```python
from build123d import *

# Parameters (mm, degrees)
ESQUISSE1_W                = 250
ESQUISSE1_H                = 50
BOSS_EXTRU_1_DEPTH         = 3.175
ESQUISSE2_W                = 10
ESQUISSE2_H                = 3.175
BOSS_EXTRU_2_DEPTH         = 3.175
R_P_TITION_LIN_AIRE1_COUNT = 13
R_P_TITION_LIN_AIRE1_PITCH = 20
ESQUISSE4_W                = 40
ESQUISSE4_H                = 23
ESQUISSE4_W_2              = 20
ESQUISSE4_H_2              = 3.175
ENL_V_MAT_EXTRU_1_DEPTH    = 3.175
ESQUISSE5_W                = 3.175
ESQUISSE5_H                = 10
BOSS_EXTRU_3_DEPTH         = 3.175
R_P_TITION_LIN_AIRE2_COUNT = 3
R_P_TITION_LIN_AIRE2_PITCH = 20
ESQUISSE6_R                = 2.18
ENL_V_MAT_EXTRU_2_DEPTH    = 10


with BuildPart() as part:
    # Esquisse1 → Boss.-Extru.1 (new body)
    with BuildSketch(Plane(origin=(0, 0, 0), x_dir=(0, 0, -1), z_dir=(1, 0, 0))):
        with Locations((125, 25)):
            Rectangle(ESQUISSE1_W, ESQUISSE1_H)
    extrude(amount=BOSS_EXTRU_1_DEPTH)

    # Esquisse2 → Boss.-Extru.2 (add)
    with BuildSketch(Plane(origin=(3.175, 0, 0), x_dir=(0, 0, -1), z_dir=(1, 0, 0))):
        with Locations((5, -1.5875)):
            Rectangle(ESQUISSE2_W, ESQUISSE2_H)
    boss_extru_2 = extrude(amount=-BOSS_EXTRU_2_DEPTH)

    # Répétition linéaire1: Boss.-Extru.2 ×13
    with Locations(*[(0, 0, -i * R_P_TITION_LIN_AIRE1_PITCH) for i in range(1, R_P_TITION_LIN_AIRE1_COUNT)]):
        add(boss_extru_2)

    # Esquisse4 → Enlèv. mat.-Extru.1 (cut)
    with BuildSketch(Plane(origin=(3.175, 0, 0), x_dir=(0, 0, -1), z_dir=(1, 0, 0))):
        with Locations((50, 8.325)):
            Rectangle(ESQUISSE4_W, ESQUISSE4_H)
        with Locations((200, 8.325)):
            Rectangle(ESQUISSE4_W, ESQUISSE4_H)
        with Locations((80, 48.4125)):
            Rectangle(ESQUISSE4_W_2, ESQUISSE4_H_2)
        with Locations((170, 48.4125)):
            Rectangle(ESQUISSE4_W_2, ESQUISSE4_H_2)
    extrude(amount=-ENL_V_MAT_EXTRU_1_DEPTH, mode=Mode.SUBTRACT)

    # Esquisse5 → Boss.-Extru.3 (add)
    with BuildSketch(Plane(origin=(3.175, 0, 0), x_dir=(0, 0, -1), z_dir=(1, 0, 0))):
        with Locations((-1.5875, 45)):
            Rectangle(ESQUISSE5_W, ESQUISSE5_H)
        with Locations((251.5875, 45)):
            Rectangle(ESQUISSE5_W, ESQUISSE5_H)
    boss_extru_3 = extrude(amount=-BOSS_EXTRU_3_DEPTH)

    # Répétition linéaire2: Boss.-Extru.3 ×3
    with Locations(*[(0, -i * R_P_TITION_LIN_AIRE2_PITCH, 0) for i in range(1, R_P_TITION_LIN_AIRE2_COUNT)]):
        add(boss_extru_3)

    # Esquisse6 → Enlèv. mat.-Extru.2 (cut)
    with BuildSketch(Plane(origin=(3.175, 0, 0), x_dir=(0, 0, -1), z_dir=(1, 0, 0))):
        with Locations((73.81, 14.99)):
            Circle(ESQUISSE6_R)
        with Locations((73.81, 4.83)):
            Circle(ESQUISSE6_R)
        with Locations((26.19, 14.99)):
            Circle(ESQUISSE6_R)
        with Locations((26.19, 4.83)):
            Circle(ESQUISSE6_R)
        with Locations((176.19, 14.99)):
            Circle(ESQUISSE6_R)
        with Locations((176.19, 4.83)):
            Circle(ESQUISSE6_R)
        with Locations((223.81, 4.83)):
            Circle(ESQUISSE6_R)
        with Locations((223.81, 14.99)):
            Circle(ESQUISSE6_R)
    extrude(amount=-ENL_V_MAT_EXTRU_2_DEPTH, mode=Mode.SUBTRACT)


solid = part.part
```
The model under review builds one solid part; all positions refer to its coordinate system, in mm. Coordinates: 2 decimals unless noted, no trailing zeros. Write each loop counter-clockwise with the first axis right and the second up, starting at its lowest first coordinate (ties: lowest second). Pieces come first, ordered by that corner, then holes. Notation, with made-up numbers: (48, 21) - (100, 21) arc R19 cw to (100, 36) - close; hole circle Ø11 at (-31.75, 9.25). An arc over 180 degrees is marked (long way). Answer in a Markdown table with one row per item. Add a question column.
Q1. Consider section A-A on y = 14.99. Give the boundary of the cut face in (x, z) (3 decimals).
Q2. Draft analysis for pull direction Z (two halves, no side actions). For faces 1 (the face through (0, 30, -123)), 2 (the face through (1.61, 15.086, -174.012)), state which applies: +Z half, -Z half, draft (parallel to the pull), parting line (faces both ways), or undercut.
Q3. Clearance check with flat-ended pins moving along their axes: pin 1 (1.6 mm diameter, centred on x = 1, y = -2.5, fed in from +Z); pin 2 (4 mm diameter, centred on y = 14.99, z = -26.19, fed in from -X); pin 3 (1.6 mm diameter, centred on x = 2, y = -1.5, fed in from -Z); pin 4 (1 mm diameter, centred on x = 1.5, z = -46, fed in from -Y) (3 decimals). State where each tip first meets the part, or that it passes through.
Q4. To check wall thickness, follow line 1 along Y through (x, z) = (1.75, -176.19) (3 decimals); line 2 along Y through (x, z) = (1.55, -223.81) (3 decimals); line 3 along Y through (x, z) = (1.2, -204.5) (3 decimals). State the ranges of each line that lie inside material, in increasing order. Write a range as from..to.
Q5. Consider section D-D on z = -73.81. Give the boundary of the cut face in (x, y) (3 decimals), then the cut area to 3 significant figures.
Q6. Consider section C-C on y = 4.83. Give the boundary of the cut face in (x, z) (3 decimals), then the cut area to 3 significant figures.
Q7. Consider section B-B on z = -223.81. Give the boundary of the cut face in (x, y) (3 decimals).
Answers below:
| question | item | result |
|---|---|---|
| 1 | outline | (0, -250) - (3.175, -250) - (3.175, -225.99) - (0, -225.99) - close; (0, -221.63) - (3.175, -221.63) - (3.175, -220) - (0, -220) - close; (0, -180) - (3.175, -180) - (3.175, -178.37) - (0, -178.37) - close; (0, -174.01) - (3.175, -174.01) - (3.175, -75.99) - (0, -75.99) - close; (0, -71.63) - (3.175, -71.63) - (3.175, -70) - (0, -70) - close; (0, -30) - (3.175, -30) - (3.175, -28.37) - (0, -28.37) - close; (0, -24.01) - (3.175, -24.01) - (3.175, 0) - (0, 0) - close |
| 2 | face 1 | draft |
| 2 | face 2 | undercut |
| 3 | pin 1 | z = 0 |
| 3 | pin 2 | through |
| 3 | pin 3 | z = -250 |
| 3 | pin 4 | y = 19.825 |
| 4 | line 1 | 0..2.65, 7.01..12.81, 17.17..46.825 |
| 4 | line 2 | -3.175..2.65, 7.01..12.81, 17.17..50 |
| 4 | line 3 | 19.825..50 |
| 5 | outline | (0, 0) - (3.175, 0) - (3.175, 2.65) - (0, 2.65) - close; (0, 7.01) - (3.175, 7.01) - (3.175, 12.81) - (0, 12.81) - close; (0, 17.17) - (3.175, 17.17) - (3.175, 46.825) - (0, 46.825) - close |
| 5 | area | 121 mm² |
| 6 | outline | (0, -253.175) - (3.175, -253.175) - (3.175, -225.99) - (0, -225.99) - close; (0, -221.63) - (3.175, -221.63) - (3.175, -220) - (0, -220) - close; (0, -180) - (3.175, -180) - (3.175, -178.37) - (0, -178.37) - close; (0, -174.01) - (3.175, -174.01) - (3.175, -75.99) - (0, -75.99) - close; (0, -71.63) - (3.175, -71.63) - (3.175, -70) - (0, -70) - close; (0, -30) - (3.175, -30) - (3.175, -28.37) - (0, -28.37) - close; (0, -24.01) - (3.175, -24.01) - (3.175, 3.175) - (0, 3.175) - close |
| 6 | area | 505 mm² |
| 7 | outline | (0, -3.175) - (3.175, -3.175) - (3.175, 2.65) - (0, 2.65) - close; (0, 7.01) - (3.175, 7.01) - (3.175, 12.81) - (0, 12.81) - close; (0, 17.17) - (3.175, 17.17) - (3.175, 50) - (0, 50) - close |
